CAD build for the part. Positions are in the model's coordinates, mm. A direction names the side the tool comes from. Coordinates: 2 decimals unless noted, no trailing zeros. Loops run counter-clockwise (first coordinate to the right, second up) from the corner with the lowest first, then second, coordinate; pieces in that order, holes last. Notation, with made-up numbers: M -9,-25.5 L 2,-25.5 A12 cw 2,-14.5 Z; hole C 24,8.5 d8. An arc over 180 degrees is marked long. Answer as a JSON object with one key per item and string values. Group by question number.
```python
from build123d import *

# Parameters (mm, degrees)
SKETCH1_R           = 60
SKETCH1_R_2         = 50
BOSS_EXTRUDE1_DEPTH = 8
SKETCH2_R           = 70
SKETCH2_R_2         = 60
BOSS_EXTRUDE2_DEPTH = 29
SKETCH3_R           = 1.5
CUT_EXTRUDE2_DEPTH  = 37
SKETCH4_R           = 2.75
CUT_EXTRUDE3_DEPTH  = 3
CIRPATTERN1_COUNT   = 6
BOSS_EXTRUDE3_START = 8
SKETCH7_R           = 70
SKETCH7_R_2         = 60
SKETCH7_R_3         = 2.75
BOSS_EXTRUDE3_DEPTH = 8


with BuildPart() as part:
    # Sketch1 → Boss-Extrude1 (new body)
    with BuildSketch(Plane.XY):
        Circle(SKETCH1_R)
        Circle(SKETCH1_R_2, mode=Mode.SUBTRACT)
    extrude(amount=BOSS_EXTRUDE1_DEPTH)



with BuildPart() as body_2:
    # Sketch2 → Boss-Extrude2 (new body)
    with BuildSketch(Plane.XY.offset(8)):
        with Locations(Location((0, 0, 0), (0, 0, 180))):
            Circle(SKETCH2_R)
        Circle(SKETCH2_R_2, mode=Mode.SUBTRACT)
    extrude(amount=BOSS_EXTRUDE2_DEPTH)

    # Sketch3 → Cut-Extrude2 (cut)
    with BuildSketch(Plane(origin=(0, 0, 8), x_dir=(-1, 0, 0), z_dir=(0, 0, -1))):
        with Locations((0, 64)):
            Circle(SKETCH3_R)
    cut_extrude2 = extrude(amount=-CUT_EXTRUDE2_DEPTH, mode=Mode.SUBTRACT)

    # Sketch4 → Cut-Extrude3 (cut)
    with BuildSketch(Plane(origin=(0, 0, 8), x_dir=(-1, 0, 0), z_dir=(0, 0, -1))):
        with Locations((0, 64)):
            Circle(SKETCH4_R)
    cut_extrude3 = extrude(amount=-CUT_EXTRUDE3_DEPTH, mode=Mode.SUBTRACT)

    # CirPattern1: Cut-Extrude2, Cut-Extrude3 ×6 about axis
    cirpattern1_axis = Axis((0, 0, 0), (0, 0, 1))
    add([cut_extrude2.rotate(cirpattern1_axis, i * 360 / CIRPATTERN1_COUNT) for i in range(1, CIRPATTERN1_COUNT)], mode=Mode.SUBTRACT)
    add([cut_extrude3.rotate(cirpattern1_axis, i * 360 / CIRPATTERN1_COUNT) for i in range(1, CIRPATTERN1_COUNT)], mode=Mode.SUBTRACT)


with BuildPart() as part_1:
    add(part.part)

    add(body_2.part)  # Boss-Extrude3 merges body 2
    # Sketch7 → Boss-Extrude3 (add)
    with BuildSketch(Plane(origin=(0, 0, 8), x_dir=(-1, 0, 0), z_dir=(0, 0, -1)).offset(BOSS_EXTRUDE3_START)):
        with Locations(Location((0, 0, 0), (0, 0, 180))):
            Circle(SKETCH7_R)
        Circle(SKETCH7_R_2, mode=Mode.SUBTRACT)
        with Locations((0, 64)):
            Circle(SKETCH7_R_3, mode=Mode.SUBTRACT)
        with Locations(Location((-55.425625842, 32, 0), (0, 0, 60))):
            Circle(SKETCH7_R_3, mode=Mode.SUBTRACT)
        with Locations(Location((-55.425625842, -32, 0), (0, 0, 120))):
            Circle(SKETCH7_R_3, mode=Mode.SUBTRACT)
        with Locations(Location((0, -64, 0), (0, 0, 180))):
            Circle(SKETCH7_R_3, mode=Mode.SUBTRACT)
        with Locations(Location((55.425625842, -32, 0), (0, 0, 240))):
            Circle(SKETCH7_R_3, mode=Mode.SUBTRACT)
        with Locations(Location((55.425625842, 32, 0), (0, 0, 300))):
            Circle(SKETCH7_R_3, mode=Mode.SUBTRACT)
    extrude(amount=-BOSS_EXTRUDE3_DEPTH)


solid = part_1.part
```
Item 1: Slice it at C-C, the plane y = 24. Write the cut outline in (x, z).
Item 2: Tool access for faces 3 (the cylindrical face through (47.69, 15.02, 3.94)), 4 (the flat face through (-23, 45, 8)), 5 (the flat face through (53.8, 32.4, 11)): list every direction of +Z, -Z, +X, -X, +Y, -Y with a clear straight run to the whole face (end or side of a thin tool).
Item 3: Slice it at B-B, the plane z = 17. Write the cut outline in (x, y).
Item 4: Slice it at A-A, the plane x = -7. Write the cut outline in (y, z).
Item 5: Drill centre lines: L1, parallel to Y at x = 0, z = 4; L2, parallel to Y at x = 0, z = 20; L3, parallel to Y at x = -43, z = 13.5. Where is each one in solid material? Low to high. Write a range as from..to.
Item 6: Pin check, flat tips, straight feed: pin 1 (4 mm diameter, centred on y = 11.5, z = 24, fed in from -X); pin 2 (4 mm diameter, centred on x = 13, z = 18, fed in from -Y); pin 3 (5 mm diameter, centred on x = 55.43, y = -32, fed in from -Z). Stop position of each tip, or through.
Item 7: Pull direction X, two halves, no side cores. Call faces 1 (the flat face through (-1.2, 62.8, 11)), 2 (the flat face through (-31, -52, 37)): released by +X, released by -X, zero draft, split by the parting line, or undercut.
Computed:
{
 "1": {"outline": "M -65.76,0 L -43.86,0 L -43.86,8 L -54.99,8 L -54.99,37 L -65.76,37 Z; M 43.86,0 L 65.76,0 L 65.76,37 L 54.99,37 L 54.99,8 L 43.86,8 Z"},
 "2": {"face 3": "+Z, -Z", "face 4": "+Z", "face 5": "-Z"},
 "3": {"outline": "C 0,0 d140; hole C 0,0 d120; hole C -55.43,-32 d3; hole C -55.43,32 d3; hole C 0,-64 d3; hole C 0,64 d3; hole C 55.43,-32 d3; hole C 55.43,32 d3"},
 "4": {"outline": "M -69.65,0 L -49.51,0 L -49.51,8 L -59.59,8 L -59.59,37 L -69.65,37 Z; M 49.51,0 L 69.65,0 L 69.65,37 L 59.59,37 L 59.59,8 L 49.51,8 Z"},
 "5": {"L1": "-70..-66.75, -61.25..-50, 50..61.25, 66.75..70", "L2": "-70..-65.5, -62.5..-60, 60..62.5, 65.5..70", "L3": "-55.24..-41.84, 41.84..55.24"},
 "6": {"pin 1": "x = -69.35", "pin 2": "y = -69.13", "pin 3": "z = 11"},
 "7": {"face 1": "undercut", "face 2": "zero draft"}
}
